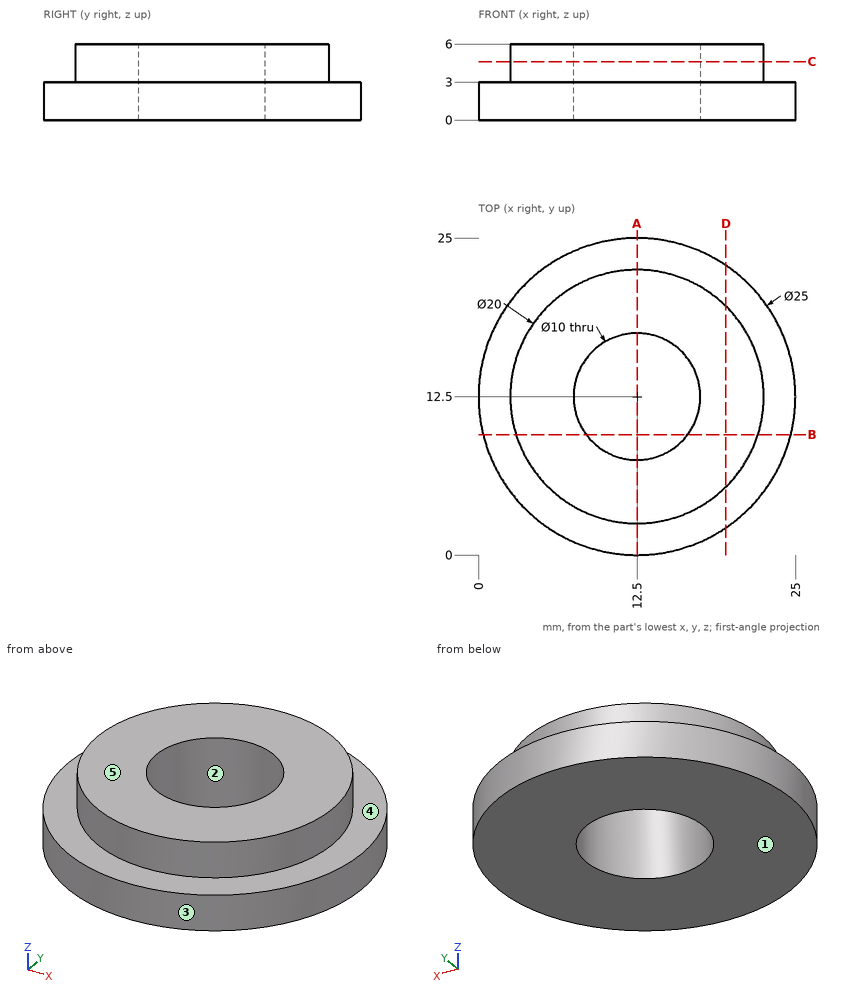
Print and shaded views of the part. All mm, measured from the part's lowest x, y and z. A direction names the side the tool comes from. Give positions to 0.01 mm unless a question says otherwise; leave off trailing zeros. Loops run counter-clockwise (first coordinate to the right, second up) from the corner with the lowest first, then second, coordinate; pieces in that order, holes last. Notation, with made-up numbers: (85, 49.25) -> (120, 49.25) arc R25 cw to (120, 70.25) -> close; hole circle Ø7 at (57.5, 52). An arc over 180 degrees is marked (long way). Use a Markdown table: item, result.
1. Mould opens along Y. For the marked faces 1, 2 and 3 say: pulls with the +Y half, pulls with the -Y half, needs draft (parallel to the pull), parting line crosses it, or undercut.
Check result:
| item | result |
|---|---|
| face 1 | needs draft |
| face 2 | undercut |
| face 3 | parting line crosses it |
2. Slice it at C-C (z = 4.6). List the corners of the cut face in (x, y).
Check result:
| item | result |
|---|---|
| outline | circle Ø20 at (12.5, 12.5); hole circle Ø10 at (12.5, 12.5) |
3. Slice it at D-D (x = 19.5). List the corners of the cut face in (y, z), plus the area to 3 significant figures.
Check result:
| item | result |
|---|---|
| outline | (2.14, 0) -> (22.86, 0) -> (22.86, 3) -> (19.64, 3) -> (19.64, 6) -> (5.36, 6) -> (5.36, 3) -> (2.14, 3) -> close |
| area | 105 mm^2 |
4. Flat gauge pins, fed straight in: pin 1 (12.5 mm diameter, centred on x = 10.5, y = 12, fed in from +Z); pin 2 (4 mm diameter, centred on x = 13, y = 14.5, fed in from +Z); pin 3 (3 mm diameter, centred on y = 19, z = 3.5, fed in from +X); pin 4 (1 mm diameter, centred on y = 8, z = 0.5, fed in from +X). Where does each tip first touch, or does it go through?
Check result:
| item | result |
|---|---|
| pin 1 | stops at z = 6 |
| pin 2 | passes through |
| pin 3 | stops at x = 23.92 |
| pin 4 | stops at x = 24.34 |
5. Which spindle directions (+Z, -Z, +X, -X, +Y, -Y) get a long thin tool onto all of the face, cutting with end or side? Do the marked faces 4 and 5. Say none if no direction does.
Check result:
| item | result |
|---|---|
| face 4 | +Z |
| face 5 | +Z, +X, -X, +Y, -Y |
6. Slice it at A-A (x = 12.5). List the corners of the cut face in (y, z), plus the area to 3 significant figures.
Check result:
| item | result |
|---|---|
| outline | (0, 0) -> (7.5, 0) -> (7.5, 6) -> (2.5, 6) -> (2.5, 3) -> (0, 3) -> close; (17.5, 0) -> (25, 0) -> (25, 3) -> (22.5, 3) -> (22.5, 6) -> (17.5, 6) -> close |
| area | 75.0 mm^2 |
7. Wall check: L1, parallel to Z at x = 3.25, y = 19; L2, parallel to Y at x = 16.25, z = 4.1; L3, parallel to Y at x = 13, z = 1.9. Give the ranges that are in metal, low to high. Write a range as [from, to].
Check result:
| item | result |
|---|---|
| L1 | z = [0, 3] |
| L2 | y = [3.23, 9.19], [15.81, 21.77] |
| L3 | y = [0.01, 7.53], [17.47, 24.99] |
8. Slice it at B-B (y = 9.5). List the corners of the cut face in (x, z), plus the area to 3 significant figures.
Check result:
| item | result |
|---|---|
| outline | (0.37, 0) -> (8.5, 0) -> (8.5, 6) -> (2.96, 6) -> (2.96, 3) -> (0.37, 3) -> close; (16.5, 0) -> (24.63, 0) -> (24.63, 3) -> (22.04, 3) -> (22.04, 6) -> (16.5, 6) -> close |
| area | 82.0 mm^2 |
